Geometry: final body of the model. Coordinates: model frame, mm. A direction names the side the tool comes from. Round coordinates to 2 decimals unless told otherwise and drop trailing zeros. Loops run counter-clockwise (first coordinate to the right, second up) from the corner with the lowest first, then second, coordinate; pieces in that order, holes last. Notation, with made-up numbers: (31.25, -12.75) - (88.25, -12.75) arc R18 ccw to (88.25, 10.25) - close; hole circle Ø2 at (6.25, 57). An arc over 180 degrees is marked (long way). Answer as CSV lines item,"result".
from build123d import *

# Parameters (mm, degrees)
SKETCH1_W                       = 100
SKETCH1_H                       = 15
BOSS_EXTRUDE1_DEPTH             = 5
M5X0_8_TAPPED_HOLE1_D           = 4.2
M5X0_8_TAPPED_HOLE1_DEPTH       = 12.4
M5X0_8_TAPPED_HOLE1_CSINK_D     = 6
M5X0_8_TAPPED_HOLE1_CSINK_ANGLE = 90
M5X0_8_TAPPED_HOLE1_TIP         = 1.2618073
SKETCH6_R                       = 5.5499
CUT_EXTRUDE1_DEPTH              = 52.53882032
CUT_EXTRUDE2_START              = -3
SKETCH7_W                       = 17.5
SKETCH7_H                       = 15
CUT_EXTRUDE2_DEPTH              = 49.53882032


with BuildPart() as part:
    # Sketch1 → Boss-Extrude1 (new, symmetric)
    with BuildSketch(Plane.XY):
        Rectangle(SKETCH1_W, SKETCH1_H)
    extrude(amount=BOSS_EXTRUDE1_DEPTH, both=True)

    # M5x0.8 Tapped Hole1
    with Locations(Plane.XY.offset(5)):
        with Locations((-28.2845, 0), (28.2845, 0)):
            CounterSinkHole(M5X0_8_TAPPED_HOLE1_D / 2, M5X0_8_TAPPED_HOLE1_CSINK_D / 2, depth=M5X0_8_TAPPED_HOLE1_DEPTH, counter_sink_angle=M5X0_8_TAPPED_HOLE1_CSINK_ANGLE)
            with Locations((0, 0, -(M5X0_8_TAPPED_HOLE1_DEPTH + M5X0_8_TAPPED_HOLE1_TIP / 2))):  # 118° drill point
                Cone(0, M5X0_8_TAPPED_HOLE1_D / 2, M5X0_8_TAPPED_HOLE1_TIP, mode=Mode.SUBTRACT)

    # Sketch6 → Cut-Extrude1 (cut, through all)
    with BuildSketch(Plane(origin=(0, 0, -5), x_dir=(-1, 0, 0), z_dir=(0, 0, -1))):
        with Locations((40, 0)):
            Circle(SKETCH6_R)
    cut_extrude1 = extrude(amount=-CUT_EXTRUDE1_DEPTH, mode=Mode.SUBTRACT)

    # Sketch7 → Cut-Extrude2 (cut, through all)
    with BuildSketch(Plane(origin=(0, 0, -5), x_dir=(-1, 0, 0), z_dir=(0, 0, -1)).offset(CUT_EXTRUDE2_START)):
        with Locations((41.25, 0)):
            Rectangle(SKETCH7_W, SKETCH7_H)
    cut_extrude2 = extrude(amount=-CUT_EXTRUDE2_DEPTH, mode=Mode.SUBTRACT)

    # Mirror1: Cut-Extrude1, Cut-Extrude2 across plane
    add(cut_extrude1.mirror(Plane(origin=(0, 0, 0), x_dir=(0, 0, 1), z_dir=(1, 0, 0))), mode=Mode.SUBTRACT)
    add(cut_extrude2.mirror(Plane(origin=(0, 0, 0), x_dir=(0, 0, 1), z_dir=(1, 0, 0))), mode=Mode.SUBTRACT)


solid = part.part
(1) Section B-B (y = 0). Output: boundary loops of the cut face in (x, z), and give its area (3 significant figures).
Findings below:
outline,"(-50, -5) - (-45.55, -5) - (-45.55, -2) - (-50, -2) - close; (-34.45, -5) - (-30.38, -5) - (-30.38, 4.1) - (-31.28, 5) - (-32.5, 5) - (-32.5, -2) - (-34.45, -2) - close; (-26.18, -5) - (26.18, -5) - (26.18, 4.1) - (25.28, 5) - (-25.28, 5) - (-26.18, 4.1) - close; (30.38, -5) - (34.45, -5) - (34.45, -2) - (32.5, -2) - (32.5, 5) - (31.28, 5) - (30.38, 4.1) - close; (45.55, -5) - (50, -5) - (50, -2) - (45.55, -2) - close"
area,"603 mm2"
(2) Pin query (flat end, axial travel): P1, Ø5, axis at y = -4.5, z = 1, coming from the -X side; P2, Ø1, axis at y = -1.5, z = 2.5, coming from the +X side; P3, Ø7.5, axis at x = -41, y = 3.5, coming from the +Z side. Return the tip coordinate at first contact, or that it passes through.
Findings below:
P1,"x = -32.5"
P2,"x = 32.5"
P3,"z = -2"
(3) Access query for faces 4 (the face through (-26.187, 0.092, -0.514)), 5 (the face through (32.5, 0, 1)), 6 (the face through (-32.5, 0, 1)). Directions: +Z, -Z, +X, -X, +Y, -Y. A direction counts if a zero-diameter tool reaches every point of the face in a straight line with its end or side. Return the directions, or none.
Findings below:
face 4,"+Z, -Z"
face 5,"+Z, +X, +Y, -Y"
face 6,"+Z, -X, +Y, -Y"
(4) Material intervals for line 1 along X through (y, z) = (-1.25, 0.25); line 2 along X through (y, z) = (0, 1.75); line 3 along Y through (x, z) = (40, -3.95), sorted ascending.
Findings below:
line 1,"-32.5 to -29.97, -26.6 to 26.6, 29.97 to 32.5"
line 2,"-32.5 to -30.38, -26.18 to 26.18, 30.38 to 32.5"
line 3,"-7.5 to -5.55, 5.55 to 7.5"
(5) Section D-D (y = -4). Output: boundary loops of the cut face in (x, z).
Findings below:
outline,"(-50, -5) - (-43.85, -5) - (-43.85, -2) - (-50, -2) - close; (-36.15, -5) - (36.15, -5) - (36.15, -2) - (32.5, -2) - (32.5, 5) - (-32.5, 5) - (-32.5, -2) - (-36.15, -2) - close; (43.85, -5) - (50, -5) - (50, -2) - (43.85, -2) - close"
(6) Section A-A (x = 40). Output: boundary loops of the cut face in (y, z).
Findings below:
outline,"(-7.5, -5) - (-5.55, -5) - (-5.55, -2) - (-7.5, -2) - close; (5.55, -5) - (7.5, -5) - (7.5, -2) - (5.55, -2) - close"
(7) Draft query along X for faces 1 (the face through (-50, 0, -3)), 2 (the face through (-1, 0, -5)), 3 (the face through (26.28, 0.63, -0.51)). Return one class per face: pulls with the +X half, pulls with the -X half, needs draft (parallel to the pull), parting line crosses it, or undercut.
Findings below:
face 1,"pulls with the -X half"
face 2,"needs draft"
face 3,"undercut"
(8) Section C-C (z = -3.5). Output: boundary loops of the cut face in (x, y), and give its area (3 significant figures).
Findings below:
outline,"(-50, -7.5) - (50, -7.5) - (50, 7.5) - (-50, 7.5) - close; hole circle Ø11.1 at (-40, 0); hole circle Ø4.2 at (-28.28, 0); hole circle Ø4.2 at (28.28, 0); hole circle Ø11.1 at (40, 0)"
area,"1,280 mm2"
